Here's how the part is built. I have some questions about the finished solid (model axes, mm). Face numbers are marked on the shaded views. Coordinates: 2 decimals unless noted, no trailing zeros. Order: outer loops, then holes, each group sorted by start corner. A loop starts at its lowest first (then second) coordinate and runs counter-clockwise, first axis right, second up. Notation, with made-up numbers: (65, -11) - (119, -11) arc R37 ccw to (119, 27) - close; hole circle Ø2 at (-28.5, -2). An arc over 180 degrees is marked (long way). Answer in a Markdown table with one row per item. Add a question column.
Item 1: Will these pins go through, and if not, where does the flat tip stop? pin 1 Ø1.2 at (y, z) = (2, 16.5) entering from +X; pin 2 Ø1.5 at (y, z) = (1, 14) entering from -X.
Item 2: I want a section at D-D (x = 7). Please give me the cut outline in (y, z).
Item 3: I want a section at B-B (x = 0). Please give me the cut outline in (y, z), plus the area to 3 significant figures.
Item 4: I want a section at C-C (y = 2.1). Please give me the cut outline in (x, z), plus the area to 3 significant figures.
Item 5: I want a section at A-A (z = 15). Please give me the cut outline in (x, y).
Item 6: Thinking about a two-plate mould opening in Z: for the marked faces 1, 2 and 3, which applies, +Z half, -Z half, draft (parallel to the pull), parting line (faces both ways), or undercut?
Item 7: If I drill on line 1 along Z through (x, y) = (0, 1.45); line 2 along X through (y, z) = (0.6, -15), over which ranges is the centre line in solid material (lowest first)? Write a range as from..to.
```python
from build123d import *

# Parameters (mm, degrees)
SKETCH1_R            = 8
BOSS_EXTRUDE1_DEPTH  = 3
M2_CLEARANCE_HOLE1_D = 2.4
FILLET1_R            = 5
FILLET2_R            = 1


with BuildPart() as part:
    # Sketch1 → Boss-Extrude1 (new body)
    with BuildSketch(Plane(origin=(0, 0, 0), x_dir=(1, 0, 0), z_dir=(0, 1, 0))):
        with BuildLine():
            Line((-3.75, 18), (3.75, 18))
            Line((3.75, 18), (3.75, 11.399013115))
            ThreePointArc((3.75, 11.399013115), (12, 0), (3.75, -11.399013115))
            Line((3.75, -11.399013115), (3.75, -18))
            Line((3.75, -18), (-3.75, -18))
            Line((-3.75, -18), (-3.75, -11.399013115))
            ThreePointArc((-3.75, -11.399013115), (-12, 0), (-3.75, 11.399013115))
            Line((-3.75, 11.399013115), (-3.75, 18))
        make_face()
        Circle(SKETCH1_R, mode=Mode.SUBTRACT)
    extrude(amount=BOSS_EXTRUDE1_DEPTH)

    # M2 Clearance Hole1 (through all)
    with Locations(Plane(origin=(0, 3, 0), x_dir=(1, 0, 0), z_dir=(0, 1, 0))):
        with Locations((0, -15), (0, 15)):
            Hole(M2_CLEARANCE_HOLE1_D / 2)

    # Fillet1
    fillet1_edges = [part.edges().sort_by_distance(p)[0] for p in [
        (3.75, 1.5, -11.399013115),
        (3.75, 1.5, 11.399013115),
        (-3.75, 1.5, 11.399013115),
        (-3.75, 1.5, -11.399013115),
    ]]
    fillet(fillet1_edges, radius=FILLET1_R)

    # Fillet2
    fillet2_edges = [part.edges().sort_by_distance(p)[0] for p in [
        (3.75, 1.5, 18),
        (-3.75, 1.5, 18),
        (-3.75, 1.5, -18),
        (3.75, 1.5, -18),
    ]]
    fillet(fillet2_edges, radius=FILLET2_R)


solid = part.part
```
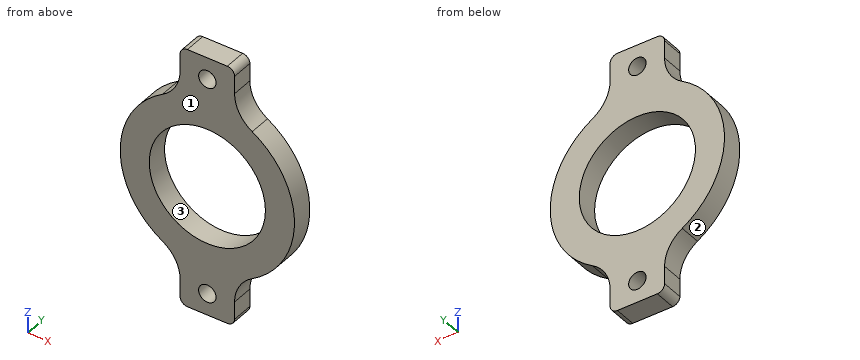
Values follow:
| question | item | result |
|---|---|---|
| 1 | pin 1 | stops at x = 3.75 |
| 1 | pin 2 | stops at x = -3.93 |
| 2 | outline | (0, -9.75) - (3, -9.75) - (3, -3.87) - (0, -3.87) - close; (0, 3.87) - (3, 3.87) - (3, 9.75) - (0, 9.75) - close |
| 3 | outline | (0, -18) - (3, -18) - (3, -16.2) - (0, -16.2) - close; (0, -13.8) - (3, -13.8) - (3, -8) - (0, -8) - close; (0, 8) - (3, 8) - (3, 13.8) - (0, 13.8) - close; (0, 16.2) - (3, 16.2) - (3, 18) - (0, 18) - close |
| 3 | area | 45.6 mm^2 |
| 4 | outline | (-6.18, -10.29) arc R5 cw to (-3.75, -14.58) - (-3.75, -17) arc R1 ccw to (-2.75, -18) - (2.75, -18) arc R1 ccw to (3.75, -17) - (3.75, -14.58) arc R5 cw to (6.18, -10.29) arc R12 ccw to (6.18, 10.29) arc R5 cw to (3.75, 14.58) - (3.75, 17) arc R1 ccw to (2.75, 18) - (-2.75, 18) arc R1 ccw to (-3.75, 17) - (-3.75, 14.58) arc R5 cw to (-6.18, 10.29) arc R12 ccw to start; hole circle Ø16 at (0, 0); hole circle Ø2.4 at (0, -15); hole circle Ø2.4 at (0, 15) |
| 4 | area | 341 mm^2 |
| 5 | outline | (-3.75, 0) - (-1.2, 0) - (-1.2, 3) - (-3.75, 3) - close; (1.2, 0) - (3.75, 0) - (3.75, 3) - (1.2, 3) - close |
| 6 | face 1 | draft |
| 6 | face 2 | parting line |
| 6 | face 3 | undercut |
| 7 | line 1 | z = -18..-16.2, -13.8..-8, 8..13.8, 16.2..18 |
| 7 | line 2 | x = -3.75..-1.2, 1.2..3.75 |
